Build history of the part. All positions in model axes, mm. A direction names the side the tool comes from. Coordinates: 2 decimals unless noted, no trailing zeros. Write each loop counter-clockwise with the first axis right and the second up, starting at its lowest first coordinate (ties: lowest second). Pieces come first, ordered by that corner, then holes. Notation, with made-up numbers: M -29.5,-14 L -15.5,-14 A24 cw -15.5,23 Z; hole C 81,32.25 d10. An arc over 180 degrees is marked long. Use CSV: the item, a comma, the result in double quotes. Start each with the question number.
```python
from build123d import *

# Parameters (mm, degrees)
SKETCH1_R           = 6
SKETCH1_R_2         = 2
BOSS_EXTRUDE1_DEPTH = 9
SKETCH2_R           = 12
SKETCH2_R_2         = 2
BOSS_EXTRUDE2_DEPTH = 5
SKETCH3_R           = 1
CUT_EXTRUDE1_DEPTH  = 7
SKETCH4_R           = 1
CUT_EXTRUDE2_DEPTH  = 5


with BuildPart() as part:
    # Sketch1 → Boss-Extrude1 (new body)
    with BuildSketch(Plane.XY):
        with Locations((-41.143471688, 10.161406423)):
            Circle(SKETCH1_R)
        with Locations((-41.143471688, 10.161406423)):
            Circle(SKETCH1_R_2, mode=Mode.SUBTRACT)
    extrude(amount=BOSS_EXTRUDE1_DEPTH)

    # Sketch2 → Boss-Extrude2 (add)
    with BuildSketch(Plane.XY.offset(9)):
        with Locations((-41.143471688, 10.161406423)):
            Circle(SKETCH2_R)
        with Locations((-41.143471688, 10.161406423)):
            Circle(SKETCH2_R_2, mode=Mode.SUBTRACT)
    extrude(amount=BOSS_EXTRUDE2_DEPTH)

    # Sketch3 → Cut-Extrude1 (cut)
    with BuildSketch(Plane(origin=(0, 17.811406423, 0), x_dir=(1, 0, 0), z_dir=(0, 1, 0))):
        with Locations(Location((-41.143471688, -5, 0), (0, 0, 180))):
            Circle(SKETCH3_R)
    extrude(amount=-CUT_EXTRUDE1_DEPTH, mode=Mode.SUBTRACT)

    # Sketch4 → Cut-Extrude2 (cut)
    with BuildSketch(Plane.XY.offset(14)):
        with Locations((-41.030441909, 18.661406423)):
            Circle(SKETCH4_R)
        with Locations((-33.838770645, 5.813519763)):
            Circle(SKETCH4_R)
        with Locations((-48.561202509, 6.009293083)):
            Circle(SKETCH4_R)
    extrude(amount=-CUT_EXTRUDE2_DEPTH, mode=Mode.SUBTRACT)


solid = part.part
```
1. 3-axis set-ups, long thin cutter, end or side, ignore diameter. For faces 4 (the flat face through (-47, 8, 9)), 5 (the cylindrical face through (-40.144, 14.057, 5.044)), 6 (the cylindrical face through (-41.58, 8.21, 6.9)): which of +Z, -Z, +X, -X, +Y, -Y reach the whole face in a straight line?
2. Slice it at C-C (z = 12.25). List the corners of the cut face in (x, y), and give its area (3 significant figures).
3. Slice it at B-B (x = -35.5). List the corners of the cut face in (y, z), and give its area (3 significant figures).
4. Drill centre lines: line 1 along Z through (x, y) = (-35, 20.25); line 2 along X through (y, z) = (6, 12.5); line 3 along X through (y, z) = (12, 10.75). Where is each one in solid material? Low to high. Write a range as from..to.
5. Slice it at A-A (y = 10.75). List the corners of the cut face in (x, z), and give its area (3 significant figures).
6. Slice it at D-D (z = 3.25). List the corners of the cut face in (x, y), and give its area (3 significant figures).
7. Pull direction X, two halves, no side cores. Call faces 1 (the flat face through (-43, 12, 0)), 2 (the cylindrical face through (-41.247, 17.685, 11.535)), 3 (the cylindrical face through (-38.37, 4.84, 4.44)): pulls with the +X half, pulls with the -X half, needs draft (parallel to the pull), parting line crosses it, or undercut.
8. Flat gauge pins, fed straight in: pin 1 (1 mm diameter, centred on x = -47.5, z = 12, fed in from -Y); pin 2 (3 mm diameter, centred on x = -50, y = 5.5, fed in from -Z); pin 3 (1 mm diameter, centred on x = -46.5, z = 2, fed in from -Y). Where does each tip first touch, or does it go through?
Established:
1,face 4,"-Z"
1,face 5,"+Y"
1,face 6,"+Z, -Z"
2,outline,"C -41.14,10.16 d24; hole C -48.56,6.01 d2; hole C -41.14,10.16 d4; hole C -41.03,18.66 d2; hole C -33.84,5.81 d2"
2,area,"430 mm2"
3,outline,"M -0.43,9 L 8.12,9 L 8.12,0 L 12.2,0 L 12.2,9 L 20.75,9 L 20.75,14 L -0.43,14 Z"
3,area,"143 mm2"
4,line 1,"z = 9..14"
4,line 2,"x = -52.4..-49.56, -47.56..-34.82, -32.86..-29.89"
4,line 3,"x = -53..-41.93, -40.36..-29.29"
5,outline,"M -53.13,9 L -47.11,9 L -47.11,0 L -43.05,0 L -43.05,14 L -53.13,14 Z; M -39.23,0 L -35.17,0 L -35.17,9 L -29.16,9 L -29.16,14 L -39.23,14 Z"
5,area,"174 mm2"
6,outline,"C -41.14,10.16 d12; hole C -41.14,10.16 d4"
6,area,"101 mm2"
7,face 1,"needs draft"
7,face 2,"undercut"
7,face 3,"parting line crosses it"
8,pin 1,"stops at y = -0.31"
8,pin 2,"stops at z = 9"
8,pin 3,"stops at y = 6.64"
